```python
from build123d import *

# Parameters (mm, degrees)
EXTRUDE002_DEPTH           = 4
EXTRUDE002_PLACEMENT_ANGLE = 180
EXTRUDE003_DEPTH           = 4
EXTRUDE003_PLACEMENT_ANGLE = 90
EXTRUDE004_DEPTH           = 4
EXTRUDE004_PLACEMENT_ANGLE = -90
EXTRUDE001_DEPTH           = 4
SKETCH_R                   = 1.75
SKETCH_R_2                 = 1.4
SKETCH_R_3                 = 2.25
EXTRUDE_DEPTH              = 5


with BuildPart() as extrude002:
    # Sketch001 → Extrude002 (new body)
    with BuildSketch(Plane.XY):
        Polygon((1.575, -7.72798), (3.15, -5), (1.575, -2.27202), (-1.575, -2.27202), (-3.15, -5), (-1.575, -7.72798), align=None)
    extrude(amount=EXTRUDE002_DEPTH)


with BuildPart() as extrude002_1:
    # Extrude002 placement: moved
    add(extrude002.part.moved(Location((0, -80, 2))).rotate(Axis((0, -80, 2), (0, 0, 1)), EXTRUDE002_PLACEMENT_ANGLE))


with BuildPart() as extrude003:
    # Sketch001 → Extrude003 (new body)
    with BuildSketch(Plane.XY):
        Polygon((1.575, -7.72798), (3.15, -5), (1.575, -2.27202), (-1.575, -2.27202), (-3.15, -5), (-1.575, -7.72798), align=None)
    extrude(amount=EXTRUDE003_DEPTH)


with BuildPart() as extrude003_1:
    # Extrude003 placement: moved
    add(extrude003.part.moved(Location((-80, 0, 2))).rotate(Axis((-80, 0, 2), (0, 0, 1)), EXTRUDE003_PLACEMENT_ANGLE))


with BuildPart() as extrude004:
    # Sketch001 → Extrude004 (new body)
    with BuildSketch(Plane.XY):
        Polygon((1.575, -7.72798), (3.15, -5), (1.575, -2.27202), (-1.575, -2.27202), (-3.15, -5), (-1.575, -7.72798), align=None)
    extrude(amount=EXTRUDE004_DEPTH)


with BuildPart() as extrude004_1:
    # Extrude004 placement: moved
    add(extrude004.part.moved(Location((80, 0, 2))).rotate(Axis((80, 0, 2), (0, 0, 1)), EXTRUDE004_PLACEMENT_ANGLE))


with BuildPart() as fusionhexnuts:
    # Sketch001 → Extrude001 (new body)
    with BuildSketch(Plane.XY):
        Polygon((1.575, -7.72798), (3.15, -5), (1.575, -2.27202), (-1.575, -2.27202), (-3.15, -5), (-1.575, -7.72798), align=None)
    extrude(amount=EXTRUDE001_DEPTH)


with BuildPart() as fusionhexnuts_1:
    # Extrude001 placement: moved
    add(fusionhexnuts.part.moved(Location((0, 80, 2))))

    # Fusion: union Extrude002, Extrude003, Extrude004
    add(extrude002_1.part)
    add(extrude003_1.part)
    add(extrude004_1.part)


with BuildPart() as cut:
    # Sketch → Extrude (new body)
    with BuildSketch(Plane.XY):
        Polygon((-5, 80), (5, 80), (80, 5), (80, -5), (63.713203, -21.286797), (84.926407, -42.5), (42.5, -84.926407), (21.286797, -63.713203), (5, -80), (-5, -80), (-80, -5), (-80, 5), (-63.713203, 21.286797), (-84.926407, 42.5), (-42.5, 84.926407), (-21.286797, 63.713203), align=None)
        with Locations((0, 75)):
            Circle(SKETCH_R, mode=Mode.SUBTRACT)
        with Locations((-75, 0)):
            Circle(SKETCH_R, mode=Mode.SUBTRACT)
        with Locations((75, 0)):
            Circle(SKETCH_R, mode=Mode.SUBTRACT)
        with Locations((0, -75)):
            Circle(SKETCH_R, mode=Mode.SUBTRACT)
        with Locations((-54.776107, 10.375)):
            Circle(SKETCH_R_2, mode=Mode.SUBTRACT)
        with Locations((-54.776107, -10.375)):
            Circle(SKETCH_R_2, mode=Mode.SUBTRACT)
        with Locations((-10.375, 54.776107)):
            Circle(SKETCH_R_2, mode=Mode.SUBTRACT)
        with Locations((10.375, 54.776107)):
            Circle(SKETCH_R_2, mode=Mode.SUBTRACT)
        with Locations((54.776107, 10.375)):
            Circle(SKETCH_R_2, mode=Mode.SUBTRACT)
        with Locations((54.776107, -10.375)):
            Circle(SKETCH_R_2, mode=Mode.SUBTRACT)
        with Locations((-10.375, -54.776107)):
            Circle(SKETCH_R_2, mode=Mode.SUBTRACT)
        with Locations((10.375, -54.776107)):
            Circle(SKETCH_R_2, mode=Mode.SUBTRACT)
        with Locations((39.244426, -63.286057)):
            Circle(SKETCH_R_2, mode=Mode.SUBTRACT)
        with Locations((63.286057, -39.244426)):
            Circle(SKETCH_R_2, mode=Mode.SUBTRACT)
        with Locations((-63.286057, 39.244426)):
            Circle(SKETCH_R_2, mode=Mode.SUBTRACT)
        with Locations((-39.244426, 63.286057)):
            Circle(SKETCH_R_2, mode=Mode.SUBTRACT)
        with Locations((-70.357125, 46.315494)):
            Circle(SKETCH_R_3, mode=Mode.SUBTRACT)
        with Locations((-46.315494, 70.357125)):
            Circle(SKETCH_R_3, mode=Mode.SUBTRACT)
        with Locations((46.315494, -70.357125)):
            Circle(SKETCH_R_3, mode=Mode.SUBTRACT)
        with Locations((70.357125, -46.315494)):
            Circle(SKETCH_R_3, mode=Mode.SUBTRACT)
        with BuildLine():
            ThreePointArc((-37.476659, -9.192388), (-47.376154, -9.192388), (-47.376154, -19.091883))
            Line((-47.376154, -19.091883), (-19.091883, -47.376154))
            ThreePointArc((-19.091883, -47.376154), (-9.192388, -47.376154), (-9.192388, -37.476659))
            Line((-37.476659, -9.192388), (-9.192388, -37.476659))
        make_face(mode=Mode.SUBTRACT)
        with BuildLine():
            ThreePointArc((19.091883, 47.376154), (9.192388, 47.376154), (9.192388, 37.476659))
            Line((9.192388, 37.476659), (37.476659, 9.192388))
            ThreePointArc((37.476659, 9.192388), (47.376154, 9.192388), (47.376154, 19.091883))
            Line((19.091883, 47.376154), (47.376154, 19.091883))
        make_face(mode=Mode.SUBTRACT)
        with BuildLine():
            ThreePointArc((-56.568542, 35.355339), (-59.39697, 35.355339), (-59.39697, 32.526912))
            Line((-59.39697, 32.526912), (-38.183766, 11.313708))
            ThreePointArc((-38.183766, 11.313708), (-35.355339, 11.313708), (-35.355339, 14.142136))
            Line((-56.568542, 35.355339), (-35.355339, 14.142136))
        make_face(mode=Mode.SUBTRACT)
        with BuildLine():
            ThreePointArc((-32.526912, 59.39697), (-35.355339, 59.39697), (-35.355339, 56.568542))
            Line((-35.355339, 56.568542), (-14.142136, 35.355339))
            ThreePointArc((-14.142136, 35.355339), (-11.313708, 35.355339), (-11.313708, 38.183766))
            Line((-32.526912, 59.39697), (-11.313708, 38.183766))
        make_face(mode=Mode.SUBTRACT)
        with BuildLine():
            ThreePointArc((14.142136, -35.355339), (11.313708, -35.355339), (11.313708, -38.183766))
            Line((11.313708, -38.183766), (32.526912, -59.39697))
            ThreePointArc((32.526912, -59.39697), (35.355339, -59.39697), (35.355339, -56.568542))
            Line((14.142136, -35.355339), (35.355339, -56.568542))
        make_face(mode=Mode.SUBTRACT)
        with BuildLine():
            ThreePointArc((56.568542, -35.355339), (59.39697, -35.355339), (59.39697, -32.526912))
            Line((59.39697, -32.526912), (38.183766, -11.313708))
            ThreePointArc((38.183766, -11.313708), (35.355339, -11.313708), (35.355339, -14.142136))
            Line((56.568542, -35.355339), (35.355339, -14.142136))
        make_face(mode=Mode.SUBTRACT)
        with BuildLine():
            ThreePointArc((3.535534, 17.67767), (-17.67767, 17.67767), (-17.67767, -3.535534))
            Line((-17.67767, -3.535534), (-3.535534, -17.67767))
            ThreePointArc((-3.535534, -17.67767), (17.67767, -17.67767), (17.67767, 3.535534))
            Line((3.535534, 17.67767), (17.67767, 3.535534))
        make_face(mode=Mode.SUBTRACT)
    extrude(amount=EXTRUDE_DEPTH)

    # Cut: cut FusionHexNuts
    add(fusionhexnuts_1.part, mode=Mode.SUBTRACT)


solid = cut.part
```
Geometry: final body of the model. Coordinates: model frame, mm. A direction names the side the tool comes from. Coordinates: 2 decimals unless noted, no trailing zeros. Order: outer loops, then holes, each group sorted by start corner. A loop starts at its lowest first (then second) coordinate and runs counter-clockwise, first axis right, second up. Notation, with made-up numbers: (88.25, -6.5) -> (106.25, -6.5) arc R24 ccw to (106.25, 22.5) -> close; hole circle Ø3 at (0, 11.25). An arc over 180 degrees is marked (long way). Write item = value, one per line.
(1) Cut plane B-B on z = 1.2. Count the separate pieces of the cut face and the enclosed holes in it, plus the area to 3 significant figures.
Solved:
separate_pieces = 1
enclosed_holes = 27
area = 14,500 mm²
(2) Pin query (flat end, axial travel): pin 1 Ø2 at (x, y) = (39.24, -63.29) entering from -Z; pin 2 Ø4.5 at (x, y) = (-75, 0.5) entering from +Z; pin 3 Ø1 at (y, z) = (3, 0.5) entering from +X; pin 4 Ø3 at (x, z) = (-68, 3.5) entering from -Y. Return the tip coordinate at first contact, or that it passes through.
Solved:
pin_1 = through
pin_2 = 2
pin_3 = 80
pin_4 = -18.5
(3) Cut plane A-A on x = 29.5. Return loops of the section in (y, z).
Solved:
outline = (-71.93, 0) -> (-56.37, 0) -> (-56.37, 5) -> (-71.93, 5) -> close; (-50.71, 0) -> (17.17, 0) -> (17.17, 5) -> (-50.71, 5) -> close; (36.97, 0) -> (55.5, 0) -> (55.5, 5) -> (36.97, 5) -> close
(4) Access query for faces 1 (the flat face through (-32.042, 74.468, 2.465)), 2 (the flat face through (48.94, -22.07, 2.46)), 3 (the flat face through (13, -72, 2)), 4 (the flat face through (-80, 0, 2)). Directions: +Z, -Z, +X, -X, +Y, -Y. A direction counts if a zero-diameter tool reaches every point of the face in a straight line with its end or side. Return the directions, or none.
Solved:
face_1 = +Z, -Z, +Y
face_2 = +Z, -Z
face_3 = +Z, -Z, -Y
face_4 = +Z, -Z, -X, -Y
(5) Line query: line 1 (Y direction, x = -75, z = 1.9); line 2 (Y direction, x = 0, z = 0.5); line 3 (X direction, y = 25, z = 4.65). Output: solid intervals per line, ascending.
Solved:
line_1 = -10 to -1.75, 1.75 to 10, 32.57 to 52.43
line_2 = -80 to -76.75, -73.25 to -20.3, 20.3 to 73.25, 76.75 to 80
line_3 = -67.43 to -51.87, -46.21 to 21.67, 41.47 to 60
(6) Pull-direction query (Y, two-part tool) for faces 5 (the flat face through (76.3, -1.4, 2)), 6 (the flat face through (-13, 72, 2)), 7 (the flat face through (32.042, -74.468, 2.465)), 8 (the flat face through (-24.897, 46.11, 2.465)); classes: pulls with the +Y half, pulls with the -Y half, needs draft (parallel to the pull), parting line crosses it, or undercut.
Solved:
face_5 = undercut
face_6 = pulls with the +Y half
face_7 = pulls with the -Y half
face_8 = undercut
